Can you work these out from the model? Positions are in its coordinate system, mm. A direction names the side the tool comes from. Coordinates: 2 decimals unless noted, no trailing zeros. Order: outer loops, then holes, each group sorted by start corner. A loop starts at its lowest first (then second) coordinate and runs counter-clockwise, first axis right, second up. Notation, with made-up numbers: (-3.75, 44.5) -> (20.25, 44.5) arc R8 cw to (20.25, 58.5) -> close; hole circle Ø11 at (7, -34.75). An arc over 180 degrees is marked (long way). Use a Markdown table: item, result. Add a question column.
1. We'd pull the mould along X, two halves only. Please class faces 1 (the flat face through (20, -10, -4)), 2 (the flat face through (21.5, 0, -2)), 3 (the cylindrical face through (-11.65, -0.21, -11.49)): pulls with the +X half, pulls with the -X half, needs draft (parallel to the pull), parting line crosses it, or undercut.
2. Suppose I cut it at B-B, the plane y = 11.5. State how many separate pieces and enclosed holes the cut face has, then the cut area to 3 significant figures.
3. Suppose I cut it at A-A, the plane x = 0. List the corners of the cut face in (y, z) for me, then the cut area to 3 significant figures.
4. For pin 1 Ø4.5 at (x, y) = (16.5, 6) entering from +Z; pin 2 Ø4.5 at (y, z) = (-11, -5.5) entering from +X; pin 3 Ø2 at (x, y) = (-10, -7) entering from -Z; pin 4 Ø3 at (x, y) = (-5, 6) entering from -Z, each with a flat end and sliding along its axis, tell me the tip position at first contact or that it passes through.
5. For faces 4 (the flat face through (18, 12, 2.75)), 5 (the flat face through (17, 0, 0.75)), 6 (the flat face through (14.7, -13, -5.8)), which set-ups out of +Z, -Z, +X, -X, +Y, -Y let a thin tool reach every point of the face, with its end or its side?
6. Suppose I cut it at D-D, the plane z = -9. List the corners of the cut face in (x, y) for me, then the cut area to 3 significant figures.
7. If I drill on line 1 along Y through (x, z) = (16.5, 7.5); line 2 along Y through (x, z) = (16.5, 1.5); line 3 along X through (y, z) = (-10, 1.3), over which ranges is the centre line in solid material (lowest first)? Write a range as from..to.
8. Suppose I cut it at C-C, the plane z = -1.25. List the corners of the cut face in (x, y) for me, then the cut area to 3 significant figures.
```python
from build123d import *

# Parameters (mm, degrees)
F1_DEPTH      = 15
F2_R          = 2
F3_DEPTH      = 14.501
F3_DEPTH_BACK = 14.501
F5_R          = 5
F6_R          = 3.5
F7_DEPTH      = 11.751
F10_DEPTH     = 11.751


with BuildPart() as f1:
    # F0 (on Front) → F1 (new body, symmetric)
    with BuildSketch(Plane.XZ):
        with BuildLine():
            ThreePointArc((12.4774797135, -0.75), (-12.5, 0), (12.4774797135, 0.75))
            Line((12.4774797135, 0.75), (21.5, 0.75))
            Line((21.5, 0.75), (21.5, 5))
            Line((21.5, 5), (10.1394673035, 12.7581116808))
            ThreePointArc((10.1394673035, 12.7581116808), (7.4511763072, 14.0546092753), (4.5, 14.5))
            Line((4.5, 14.5), (-4.5, 14.5))
            ThreePointArc((-4.5, 14.5), (-11.5710678119, 11.5710678119), (-14.5, 4.5))
            Line((-14.5, 4.5), (-14.5, -4.5))
            ThreePointArc((-14.5, -4.5), (-11.5710678119, -11.5710678119), (-4.5, -14.5))
            Line((-4.5, -14.5), (4.5, -14.5))
            ThreePointArc((4.5, -14.5), (7.4511763072, -14.0546092753), (10.1394673035, -12.7581116808))
            Line((10.1394673035, -12.7581116808), (21.5, -5))
            Line((21.5, -5), (21.5, -0.75))
            Line((21.5, -0.75), (12.4774797135, -0.75))
        make_face()
    extrude(amount=F1_DEPTH, both=True)

    # F2 (on Top) → F3 (cut, two sides)
    with BuildSketch(Plane.XY) as f3_sk:
        with Locations((16.5, 10)):
            Circle(F2_R)
        with Locations((16.5, -10)):
            Circle(F2_R)
    extrude(amount=-F3_DEPTH, mode=Mode.SUBTRACT)
    extrude(f3_sk.sketch, amount=F3_DEPTH_BACK, mode=Mode.SUBTRACT)

    # F5
    f5_edges = [f1.edges().sort_by_distance(p)[0] for p in [
        (21.5, 0, 5),
        (21.5, 0, -5),
    ]]
    fillet(f5_edges, radius=F5_R)

    # F6 (on offset) → F7 (cut, through all)
    with BuildSketch(Plane(origin=(0, 0, 2.75), x_dir=(1, 0, 0), z_dir=(0, 0, -1))):
        with Locations((16.5, 10)):
            Circle(F6_R)
        with Locations((16.5, -10)):
            Circle(F6_R)
    extrude(amount=-F7_DEPTH, mode=Mode.SUBTRACT)

    # F9 (on offset) → F10 (cut, through all)
    with BuildSketch(Plane.XY.offset(-2.75)):
        Polygon((20, 7.9792740578), (20, 12.0207259422), (16.5, 14.0414518843), (13, 12.0207259422), (13, 7.9792740578), (16.5, 5.9585481157), align=None)
        Polygon((20, -12.0207259422), (20, -7.9792740578), (16.5, -5.9585481157), (13, -7.9792740578), (13, -12.0207259422), (16.5, -14.0414518843), align=None)
    extrude(amount=-F10_DEPTH, mode=Mode.SUBTRACT)


solid = f1.part
```
Worked out:
| question | item | result |
|---|---|---|
| 1 | face 1 | undercut |
| 1 | face 2 | pulls with the +X half |
| 1 | face 3 | pulls with the -X half |
| 2 | separate pieces | 3 |
| 2 | enclosed holes | 0 |
| 2 | area | 275 mm² |
| 3 | outline | (-15, -14.5) -> (15, -14.5) -> (15, -12.5) -> (-15, -12.5) -> close; (-15, 12.5) -> (15, 12.5) -> (15, 14.5) -> (-15, 14.5) -> close |
| 3 | area | 120 mm² |
| 4 | pin 1 | stops at z = 9.95 |
| 4 | pin 2 | stops at x = 21.42 |
| 4 | pin 3 | stops at z = -13.43 |
| 4 | pin 4 | stops at z = -14.5 |
| 5 | face 4 | +Z |
| 5 | face 5 | +X, +Y, -Y |
| 5 | face 6 | -Z |
| 6 | outline | (-13.43, -15) -> (-8.67, -15) -> (-8.67, 15) -> (-13.43, 15) -> close; (8.67, -15) -> (15.64, -15) -> (15.64, -13.55) -> (13, -12.02) -> (13, -7.98) -> (15.64, -6.45) -> (15.64, 6.45) -> (13, 7.98) -> (13, 12.02) -> (15.64, 13.55) -> (15.64, 15) -> (8.67, 15) -> close |
| 6 | area | 322 mm² |
| 7 | line 1 | y = -15..-13.5, -6.5..6.5, 13.5..15 |
| 7 | line 2 | y = -15..-12, -8..8, 12..15 |
| 7 | line 3 | x = -14.5..-12.43, 12.43..14.5, 18.5..21.5 |
| 8 | outline | (-14.5, -15) -> (-12.44, -15) -> (-12.44, 15) -> (-14.5, 15) -> close; (12.44, -15) -> (21.5, -15) -> (21.5, 15) -> (12.44, 15) -> close; hole circle Ø4 at (16.5, -10); hole circle Ø4 at (16.5, 10) |
| 8 | area | 309 mm² |
